Here's the drawing with two shaded views (mm, measured from the low corner). I have some questions. A direction names the side the tool comes from. Coordinates: 2 decimals unless noted, no trailing zeros. Write each loop counter-clockwise with the first axis right and the second up, starting at its lowest first coordinate (ties: lowest second). Pieces come first, ordered by that corner, then holes. Notation, with made-up numbers: M 19.25,77 L 65.25,77 A24 cw 65.25,104 Z; hole C 5,74 d11. An arc over 180 degrees is marked long. Use one line per item in the form item = value. Start each with the question number.
1. On a 3-axis mill with a long thin cutter (end or side, diameter ignored), from which of +Z, -Z, +X, -X, +Y, -Y can I reach the whole of each face in a straight line? I mean the marked faces 4 and 5. Say none if no direction works.
2. I want a section at D-D, the plane x = 83. List the corners of the cut face in (y, z) for me.
3. Please list where these lines run through material, in increasing order: line 1 along X through (y, z) = (55, 21); line 2 along Y through (x, z) = (112.5, 43.5); line 3 along Z through (x, y) = (169, 70.5). Write a range as [from, to].
4. I want a section at B-B, the plane z = 9. List the corners of the cut face in (x, y) for me.
5. I'm going to push a flat-ended pin straight in: pin 1 Ø5 at (x, y) = (59, 47) entering from +Z. Where does the tip first touch, or does it pass through?
6. I want a section at A-A, the plane x = 42. List the corners of the cut face in (y, z) for me (1 decimal), plus the area to 3 significant figures.
7. I want a section at C-C, the plane y = 56.5. List the corners of the cut face in (x, z) for me, plus the area to 3 significant figures.
8. Thinking about a two-plate mould opening in Y: for the marked faces 1, 2 and 3, which applies, released by +Y, released by -Y, zero draft, split by the parting line, or undercut?
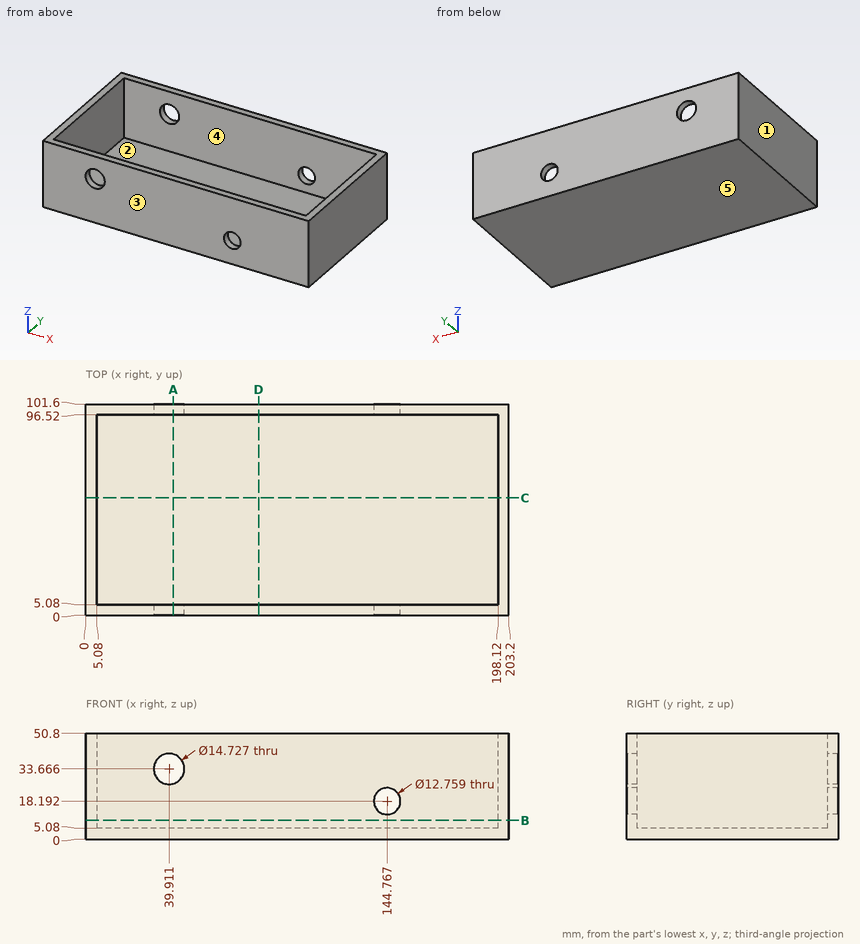
Answer list:
q1.face_4 = +Z
q1.face_5 = -Z, +X, -X, +Y, -Y
q2.outline = M 0,0 L 101.6,0 L 101.6,50.8 L 96.52,50.8 L 96.52,5.08 L 5.08,5.08 L 5.08,50.8 L 0,50.8 Z
q3.line_1 = [0, 5.08], [198.12, 203.2]
q3.line_2 = [0, 5.08], [96.52, 101.6]
q3.line_3 = [0, 5.08]
q4.outline = M 0,0 L 203.2,0 L 203.2,101.6 L 0,101.6 Z; hole M 5.08,5.08 L 198.12,5.08 L 198.12,96.52 L 5.08,96.52 Z
q5.pin_1 = 5.08
q6.outline = M 0,0 L 101.6,0 L 101.6,26.6 L 96.5,26.6 L 96.5,5.1 L 5.1,5.1 L 5.1,26.6 L 0,26.6 Z; M 0,40.7 L 5.1,40.7 L 5.1,50.8 L 0,50.8 Z; M 96.5,40.7 L 101.6,40.7 L 101.6,50.8 L 96.5,50.8 Z
q6.area = 837 mm²
q7.outline = M 0,0 L 203.2,0 L 203.2,50.8 L 198.12,50.8 L 198.12,5.08 L 5.08,5.08 L 5.08,50.8 L 0,50.8 Z
q7.area = 1,500 mm²
q8.face_1 = zero draft
q8.face_2 = undercut
q8.face_3 = released by -Y
